Can you work these out from the model? Positions are in its coordinate system, mm. Face numbers are marked on the shaded views. A direction names the side the tool comes from. Coordinates: 2 decimals unless noted, no trailing zeros. Order: outer loops, then holes, each group sorted by start corner. A loop starts at its lowest first (then second) coordinate and runs counter-clockwise, first axis right, second up. Notation, with made-up numbers: (82.5, 61) -> (92.5, 61) arc R11 ccw to (92.5, 81) -> close; hole circle Ø4 at (-25, 29.25). An arc over 180 degrees is marked (long way). Return JSON: item names as keys, results as strings. Group by question number.
1) If I drill on probe 1 along Z at (x, y) = (-14.5, 22); probe 2 along Z at (x, y) = (-30, 9.5); probe 3 along Z at (x, y) = (-45, 1.5), over which ranges is the centre line in solid material (lowest first)? Write a range as from..to.
2) Thinking about a two-plate mould opening in X: for the marked faces 1, 2 and 3, which applies, +X half, -X half, draft (parallel to the pull), parting line (faces both ways), or undercut?
3) For pin 1 (10 mm diameter, centred on x = -26, y = 24.5, fed in from +Z); pin 2 (8 mm diameter, centred on y = 20.5, z = 28, fed in from +X); pin 3 (4 mm diameter, centred on y = 1, z = 11.5, fed in from -X), each with a flat end and sliding along its axis, tell me the tip position at first contact or that it passes through.
4) If we section it at B-B, the plane x = -16.5: Please give me the cut outline in (y, z), then the cut area to 3 significant figures.
5) If we section it at A-A, the plane y = 21: Please give me the cut outline in (x, z), then the cut area to 3 significant figures.
6) If we section it at C-C, the plane z = 13.5: Please give me the cut outline in (x, y).
7) For the marked faces 4, 5, 6 and 7, which set-ups out of +Z, -Z, +X, -X, +Y, -Y let a thin tool reach every point of the face, with its end or its side?
8) If we section it at D-D, the plane y = 10.5: Please give me the cut outline in (x, z), then the cut area to 3 significant figures.
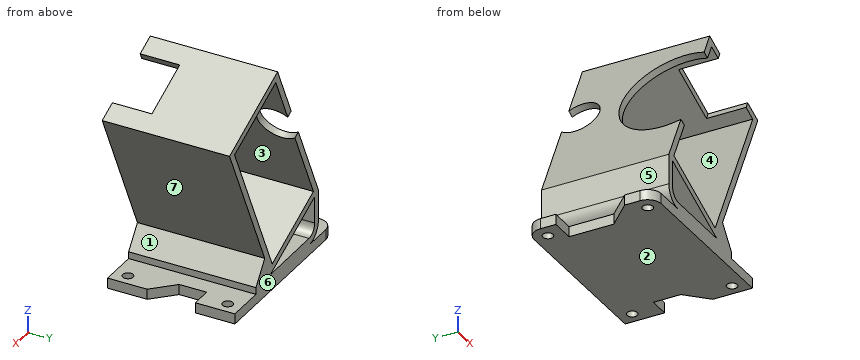
from build123d import *

# Parameters (mm, degrees)
CROQUIS1_R              = 1.5
SALIENTE_EXTRUIR1_DEPTH = 3
SALIENTE_EXTRUIR2_DEPTH = 37
CROQUIS4_R              = 15.5
CROQUIS4_R_2            = 6
CORTAR_EXTRUIR1_DEPTH   = 2
CORTAR_EXTRUIR2_DEPTH   = 2


with BuildPart() as part:
    # Croquis1 → Saliente-Extruir1 (new body)
    with BuildSketch(Plane.XY):
        with BuildLine():
            Line((-49.197309417, 11.961883408), (-56.197309417, 4.961883408))
            Line((-56.197309417, 4.961883408), (-56.197309417, 0.461883408))
            ThreePointArc((-56.197309417, 0.461883408), (-55.099110766, -2.293519818), (-52.406664651, -3.538116592))
            Line((-52.406664651, -3.538116592), (-4.197309417, -3.538116592))
            Line((-4.197309417, -3.538116592), (-4.197309417, 7.961883408))
            Line((-4.197309417, 7.961883408), (-10.197309417, 13.961883408))
            Line((-10.197309417, 13.961883408), (-10.197309417, 21.961883408))
            Line((-10.197309417, 21.961883408), (-4.197309417, 21.961883408))
            Line((-4.197309417, 21.961883408), (-4.197309417, 33.461883408))
            Line((-4.197309417, 33.461883408), (-52.197309417, 33.461883408))
            ThreePointArc((-52.197309417, 33.461883408), (-55.025736542, 32.290310533), (-56.197309417, 29.461883408))
            Line((-56.197309417, 29.461883408), (-56.197309417, 24.961883408))
            Line((-56.197309417, 24.961883408), (-49.197309417, 24.961883408))
            Line((-49.197309417, 24.961883408), (-49.197309417, 11.961883408))
        make_face()
        with Locations((-52.19152813, 0.461883408)):
            Circle(CROQUIS1_R, mode=Mode.SUBTRACT)
        with Locations((-7.69152813, 0.461883408)):
            Circle(CROQUIS1_R, mode=Mode.SUBTRACT)
        with Locations((-52.197309417, 29.461883408)):
            Circle(CROQUIS1_R, mode=Mode.SUBTRACT)
        with Locations((-7.697309417, 29.461882832)):
            Circle(CROQUIS1_R, mode=Mode.SUBTRACT)
    extrude(amount=SALIENTE_EXTRUIR1_DEPTH)

    # Croquis3 → Saliente-Extruir2 (add)
    with BuildSketch(Plane.XZ.offset(3.538116592)):
        with BuildLine():
            Line((-28.301987034, 3), (-15.301987034, 3))
            Line((-15.301987034, 3), (-15.301987034, 5))
            Line((-15.301987034, 5), (-19.967041165, 11.226302412))
            Line((-19.967041165, 11.226302412), (-1.371837648, 51.103845041))
            Line((-1.371837648, 51.103845041), (-26.748455685, 62.93715637))
            Line((-26.748455685, 62.93715637), (-48.301987034, 16.715459231))
            Line((-48.301987034, 16.715459231), (-48.301987034, 8))
            ThreePointArc((-48.301987034, 8), (-46.83752094, 4.464466094), (-43.301987034, 3))
            Line((-43.301987034, 3), (-28.301987034, 3))
        make_face()
        Polygon((-45.644134936, 17.682838282), (-25.781076635, 60.279304272), (-4.029689746, 50.136465991), (-23.892748048, 7.54), align=None, mode=Mode.SUBTRACT)
        with BuildLine():
            Line((-43.301987034, 5), (-22.925368997, 4.882147902))
            Line((-22.925368997, 4.882147902), (-46.301987034, 15.782843915))
            Line((-46.301987034, 15.782843915), (-46.301987034, 8))
            ThreePointArc((-46.301987034, 8), (-45.423307378, 5.878679656), (-43.301987034, 5))
        make_face(mode=Mode.SUBTRACT)
    extrude(amount=-SALIENTE_EXTRUIR2_DEPTH)

    # Croquis4 → Cortar-Extruir1 (cut)
    with BuildSketch(Plane(origin=(-46.07734524, 0, 21.486218953), x_dir=(0.42261826174069334, 0, 0.9063077870366529), z_dir=(-0.9063077870366529, 0, 0.42261826174069334))):
        with Locations((24.316351755, 1.961883408)):
            Circle(CROQUIS4_R)
        with Locations((24.316351755, 29.461883408)):
            Circle(CROQUIS4_R_2)
    extrude(amount=-CORTAR_EXTRUIR1_DEPTH, mode=Mode.SUBTRACT)

    # Croquis5 → Cortar-Extruir2 (cut)
    with BuildSketch(Plane(origin=(19.328889555, 0, 41.450937417), x_dir=(0.9063077870366526, 0, -0.42261826174069395), z_dir=(0.42261826174069395, 0, 0.9063077870366526))):
        Polygon((-36.840725303, -3.538116592), (-44.940725303, -3.538116592), (-44.940725303, 7.961883408), (-28.740725303, 7.961883408), (-28.740725303, -3.538116592), align=None)
    extrude(amount=-CORTAR_EXTRUIR2_DEPTH, mode=Mode.SUBTRACT)


solid = part.part
Result sheet:
{
 "1": {"probe 1": "z = 0..3, 22.95..27.68, 55.02..57.23", "probe 2": "z = 0..4.92, 8.18..10.39, 55.76..55.96", "probe 3": "z = 0..3, 3.3..5.53, 15.18..17.38, 19.06..23.8"},
 "2": {"face 1": "+X half", "face 2": "draft", "face 3": "undercut"},
 "3": {"pin 1": "stops at z = 62.94", "pin 2": "stops at x = -10.28", "pin 3": "stops at x = -48.3"},
 "4": {"outline": "(-3.54, 0) -> (33.46, 0) -> (33.46, 6.6) -> (-3.54, 6.6) -> close; (-3.54, 18.66) -> (33.46, 18.66) -> (33.46, 23.39) -> (-3.54, 23.39) -> close; (7.96, 55.95) -> (33.46, 55.95) -> (33.46, 58.16) -> (7.96, 58.16) -> close", "area": "476 mm2"},
 "5": {"outline": "(-49.2, 0) -> (-10.2, 0) -> (-10.2, 3) -> (-15.3, 3) -> (-15.3, 5) -> (-19.97, 11.23) -> (-1.37, 51.1) -> (-26.75, 62.94) -> (-48.3, 16.72) -> (-48.3, 8) arc R5 ccw to (-43.3, 3) -> (-49.2, 3) -> close; hole (-46.3, 8) arc R3 ccw to (-43.3, 5) -> (-22.93, 4.88) -> (-46.3, 15.78) -> close; hole (-45.64, 17.68) -> (-23.89, 7.54) -> (-4.03, 50.14) -> (-25.78, 60.28) -> close", "area": "524 mm2"},
 "6": {"outline": "(-48.3, -3.54) -> (-46.3, -3.54) -> (-46.3, 33.46) -> (-48.3, 33.46) -> close; (-41.41, -3.54) -> (-36.67, -3.54) -> (-36.67, 33.46) -> (-41.41, 33.46) -> close; (-21.11, -3.54) -> (-18.91, -3.54) -> (-18.91, 33.46) -> (-21.11, 33.46) -> close"},
 "7": {"face 4": "+Y, -Y", "face 5": "+Z, -X, +Y, -Y", "face 6": "+Z, -Z, +X, -X, +Y", "face 7": "+X, +Y, -Y"},
 "8": {"outline": "(-50.66, 0) -> (-6.74, 0) -> (-6.74, 3) -> (-15.3, 3) -> (-15.3, 5) -> (-19.97, 11.23) -> (-1.37, 51.1) -> (-26.75, 62.94) -> (-30.33, 55.25) -> (-28.52, 54.4) -> (-25.78, 60.28) -> (-4.03, 50.14) -> (-23.89, 7.54) -> (-45.64, 17.68) -> (-39.46, 30.95) -> (-41.27, 31.8) -> (-48.3, 16.72) -> (-48.3, 8) arc R5 ccw to (-43.3, 3) -> (-50.66, 3) -> close; hole (-46.3, 8) arc R3 ccw to (-43.3, 5) -> (-22.93, 4.88) -> (-46.3, 15.78) -> close", "area": "487 mm2"}
}
